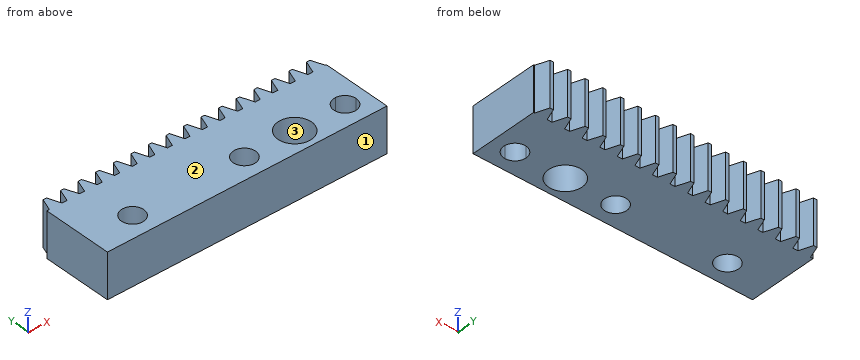
from build123d import *

# Parameters (mm, degrees)
BLANKSKE_W         = 25
BLANKSKE_H         = 7.3
BLANK_DEPTH        = 4
TOOTHCUTSIM_DEPTH  = 27.349383294
TEETHCUTS_COUNT    = 17
TEETHCUTS_PITCH    = 1.570796325
CUT_EXTRUDE1_DEPTH = 27.349383294


with BuildPart() as part:
    # BlankSke → Blank (new body)
    with BuildSketch(Plane.XY):
        with Locations((12.5, 3.65)):
            Rectangle(BLANKSKE_W, BLANKSKE_H)
    extrude(amount=-BLANK_DEPTH)

    # TooCutSkeSim → ToothCutSim (cut, through all)
    with BuildSketch(Plane.XY):
        Polygon((0.222217685, 6.175), (-0.222217685, 6.175), (-0.640929042, 7.3254), (0.640929042, 7.3254), align=None)
    toothcutsim = extrude(amount=-TOOTHCUTSIM_DEPTH, mode=Mode.SUBTRACT)

    # TeethCuts: ToothCutSim ×17
    with Locations(*[(i * TEETHCUTS_PITCH, 0, 0) for i in range(1, TEETHCUTS_COUNT)]):
        add(toothcutsim, mode=Mode.SUBTRACT)

    # Sketch1 → Cut-Extrude1 (cut, through all)
    with BuildSketch(Plane(origin=(0, 0, -4), x_dir=(-1, 0, 0), z_dir=(0, 0, -1))):
        with BuildLine():
            Line((-23, 1), (-23, 2))
            Line((-23, 2), (-24, 2))
            ThreePointArc((-24, 2), (-23.707106781, 1.292893219), (-23, 1))
        make_face()
        with BuildLine():
            Line((-24, 2), (-23, 2))
            Line((-23, 2), (-23, 3))
            ThreePointArc((-23, 3), (-23.707106781, 2.707106781), (-24, 2))
        make_face()
        with BuildLine():
            Line((-23, 3), (-23, 2))
            Line((-23, 2), (-23, 1))
            ThreePointArc((-23, 1), (-22.292893219, 1.292893219), (-22, 2))
            ThreePointArc((-22, 2), (-22.292893219, 2.707106781), (-23, 3))
        make_face()
        with BuildLine():
            ThreePointArc((-17, 2), (-18.5, 3.5), (-20, 2))
            Line((-20, 2), (-17, 2))
        make_face()
        with BuildLine():
            Line((-17, 2), (-20, 2))
            ThreePointArc((-20, 2), (-18.5, 0.5), (-17, 2))
        make_face()
        with BuildLine():
            ThreePointArc((-13, 2), (-14, 3), (-15, 2))
            Line((-15, 2), (-13, 2))
        make_face()
        with BuildLine():
            Line((-13, 2), (-15, 2))
            ThreePointArc((-15, 2), (-14, 1), (-13, 2))
        make_face()
        with BuildLine():
            ThreePointArc((-3, 2), (-4, 3), (-5, 2))
            Line((-5, 2), (-3, 2))
        make_face()
        with BuildLine():
            Line((-3, 2), (-5, 2))
            ThreePointArc((-5, 2), (-4, 1), (-3, 2))
        make_face()
    extrude(amount=-CUT_EXTRUDE1_DEPTH, mode=Mode.SUBTRACT)


solid = part.part
Source: CAD feature listing. Evaluate the final solid. Frame: model axes, mm. Face numbers are marked on the shaded views. Give positions to 0.01 mm unless a question says otherwise; leave off trailing zeros. Answer as a JSON object with one key per item and string values.
Q1. Cut plane A-A, the plane z = -0.9. Count the separate pieces of the cut face and the enclosed holes in it, then the cut area to 3 significant figures.
Geometry check:
{"separate pieces": "1", "enclosed holes": "4", "area": "151 mm^2"}
Q2. Mould query, pull axis Y, two halves, no side actions, for the marked faces 1, 2 and 3. Classes: +Y half, -Y half, draft (parallel to the pull), parting line (faces both ways), or undercut.
Geometry check:
{"face 1": "-Y half", "face 2": "draft", "face 3": "undercut"}
Q3. Contact query for a flat-ended pin moving along its axis: P1, Ø1.8, axis at x = 14, y = 2, coming from the +Z side. Output: stop coordinate, or through.
Geometry check:
{"P1": "passes through"}
Q4. Ray query, line 1 along X through (y, z) = (2, -1.15); line 2 along Y through (x, z) = (14, -0.85) (3 decimals); line 3 along X through (y, z) = (1.25, -2.6). Return the intervals inside material, ascending.
Geometry check:
{"line 1": "x = 0 to 3, 5 to 13, 15 to 17, 20 to 22, 24 to 25", "line 2": "y = 0 to 1, 3 to 6.175", "line 3": "x = 0 to 3.34, 4.66 to 13.34, 14.66 to 17.2, 19.8 to 22.34, 23.66 to 25"}
